```python
from build123d import *

# Parameters (mm, degrees)
F0_R     = 13.7
F1_DEPTH = 2.15
F2_R     = 1
F4_DEPTH = 2.15


with BuildPart() as f1:
    # F0 (on Top) → F1 (new body)
    with BuildSketch(Plane.XY):
        Circle(F0_R)
    extrude(amount=F1_DEPTH)

    # F2
    f2_edges = [f1.edges().sort_by_distance(p)[0] for p in [
        (-13.7, 0, 2.15),
        (-13.7, 0, 0),
    ]]
    fillet(f2_edges, radius=F2_R)

    # F3 (on face) → F4 (cut, through all)
    with BuildSketch(Plane(origin=(0, 0, 0), x_dir=(1, 0, 0), z_dir=(0, 0, -1))):
        Polygon((-3.3669322911, -3.197086975), (-2.673119963, -3.197086975), (-4.7889700387, -0.3285892857), (-2.749716844, 1.8749586682), (-3.4468594713, 1.8749586682), (-5.7469861014, -0.6405273085), (-5.7469861014, 1.8749586682), (-6.3364490553, 1.8749586682), (-6.3364490553, -3.197086975), (-5.7469861014, -3.197086975), (-5.7469861014, -1.2088983676), (-5.2152483331, -0.7371059845), align=None)
        with BuildLine():
            Line((1.1957695829, 0.0513130465), (0.6036887334, 0.1377061204))
            add(Edge.make_bspline(
                [(0.3380255409, -0.3335847345), (0.5428237209, -0.1592137126), (0.6036887334, 0.1377061204)],
                knots=[0, 0, 0, 0.7028049152, 0.7028049152, 0.7028049152], degree=2))
            add(Edge.make_bspline(
                [(-0.5772516823, -0.581692023), (0.0466243631, -0.581692023), (0.3380255409, -0.3335847345)],
                knots=[0, 0, 0, 1, 1, 1], degree=2))
            Line((-0.5772516823, -0.581692023), (-1.3865143818, -0.581692023))
            Line((-1.3865143818, -0.581692023), (-1.3865143818, 0.17412538))
            Line((-1.3865143818, 0.17412538), (-1.9759773358, 0.17412538))
            Line((-1.9759773358, 0.17412538), (-1.9759773358, -3.197086975))
            Line((-1.9759773358, -3.197086975), (-1.3865143818, -3.197086975))
            Line((-1.3865143818, -3.197086975), (-1.3865143818, -1.0878974976))
            Line((-1.3865143818, -1.0878974976), (-0.3274792442, -1.0878974976))
            Line((-0.3274792442, -1.0878974976), (0.9002910515, -3.197086975))
            Line((0.9002910515, -3.197086975), (1.5974336788, -3.197086975))
            Line((1.5974336788, -3.197086975), (0.2197999202, -0.9180522397))
            add(Edge.make_bspline(
                [(1.1957695829, 0.0513130465), (1.0276039433, -0.6376501903), (0.2197999202, -0.9180522397)],
                knots=[0.2081762837, 0.2081762837, 0.2081762837, 1, 1, 1], degree=2))
        make_face()
        with BuildLine():
            add(Edge.make_bspline(
                [(0.6149774989, 0.619108323), (0.5639843778, 0.9626327865), (0.3330300921, 1.1356322514)],
                knots=[0.2207931367, 0.2207931367, 0.2207931367, 1, 1, 1], degree=2))
            Line((0.6149774989, 0.619108323), (1.2327357734, 0.619108323))
            add(Edge.make_bspline(
                [(0.7942765278, 1.5175065568), (1.1831529928, 1.2056305376), (1.2327357734, 0.619108323)],
                knots=[0, 0, 0, 0.872497348, 0.872497348, 0.872497348], degree=2))
            add(Edge.make_bspline(
                [(-0.5850223804, 1.8749586682), (0.3485714883, 1.8749586682), (0.7942765278, 1.5175065568)],
                knots=[0, 0, 0, 1, 1, 1], degree=2))
            Line((-0.5850223804, 1.8749586682), (-1.9759773358, 1.8749586682))
            Line((-1.9759773358, 1.8749586682), (-1.9759773358, 0.7536415942))
            Line((-1.9759773358, 0.7536415942), (-1.3865143818, 0.7536415942))
            Line((-1.3865143818, 0.7536415942), (-1.3865143818, 1.3576521964))
            Line((-1.3865143818, 1.3576521964), (-0.6194354719, 1.3576521964))
            add(Edge.make_bspline(
                [(0.3330300921, 1.1356322514), (0.0366334655, 1.3576521964), (-0.6194354719, 1.3576521964)],
                knots=[0, 0, 0, 1, 1, 1], degree=2))
        make_face()
        with BuildLine():
            Line((3.7232746521, 1.896050563), (3.0058799547, 0.0735661382))
            Line((3.0058799547, 0.0735661382), (3.5263660581, -0.0564224731))
            Line((3.5263660581, -0.0564224731), (3.7443665468, 0.5184168044))
            add(Edge.make_bspline(
                [(3.9630561926, 1.2499725231), (3.8864593116, 0.9169426056), (3.7443665468, 0.5184168044)],
                knots=[0, 0, 0, 1, 1, 1], degree=2))
            add(Edge.make_bspline(
                [(4.1983973343, 0.5184168044), (4.0840570627, 0.8170336304), (3.9630561926, 1.2499725231)],
                knots=[0, 0, 0, 1, 1, 1], degree=2))
            Line((4.1983973343, 0.5184168044), (4.3359644272, 0.1522607828))
            Line((4.3359644272, 0.1522607828), (4.810570116, 0.3869358669))
            Line((4.810570116, 0.3869358669), (4.2194892291, 1.896050563))
            Line((4.2194892291, 1.896050563), (3.7232746521, 1.896050563))
        make_face()
        Polygon((3.3957695214, -0.40078876), (2.8680717842, -0.2765246073), (1.7184345488, -3.197086975), (2.3156682008, -3.197086975), (2.9395442462, -1.5841120746), (4.9721368426, -1.5841120746), (5.6037835861, -3.197086975), (6.2143384348, -3.197086975), (4.9638303876, -0.0043596959), (4.5097831967, -0.3103846639), (4.788970388, -1.0534844061), (3.1482429945, -1.0534844061), align=None)
    extrude(amount=-F4_DEPTH, mode=Mode.SUBTRACT)


solid = f1.part
```
Geometry: final body of the model. Coordinates: model frame, mm. A direction names the side the tool comes from. Give positions to 0.01 mm unless a question says otherwise; leave off trailing zeros.
1. Pin query (flat end, axial travel): P1, Ø0.5, axis at x = -6, z = 1.5, coming from the +Y side; P2, Ø0.8, axis at x = -1, z = 1, coming from the -Y side; P3, Ø0.7, axis at x = -1, z = 1, coming from the +Y side. Return the tip coordinate at first contact, or that it passes through.
2. Line query: probe 1 along Y at (x, z) = (1, 1.15); probe 2 along X at (y, z) = (1.25, 1.2); probe 3 along Y at (x, z) = (-0.75, 1.3). Output: solid intervals per line, ascending.
3. Reachability of faces 3 (the flat face through (-4.304, 1.95, 1.06)), 4 (the flat face through (0, 0, 2.15)) from +Z, -Z, +X, -X, +Y, -Y: full face, straight path, thin tool, end or side. Return the list, or none.
4. Draft query along Y for faces 1 (the flat face through (0, 0, 0)), 2 (the flat face through (-1, -1.875, 1)). Return one class per face: released by +Y, released by -Y, zero draft, split by the parting line, or undercut.
Computed:
1. P1: stops at y = 12.39
1. P2: stops at y = -13.69
1. P3: stops at y = 13.68
2. probe 1: y = -13.66 to -1.3, -0.62 to -0.08, 0.38 to 2.21, 3.2 to 13.66
2. probe 2: x = -13.64 to -6.34, -5.75 to -4.83, -4.11 to -1.98, -1.39 to -0.23, 0.42 to 2.48, 5.45 to 13.64
2. probe 3: y = -13.67 to -1.87, -1.36 to 0.58, 1.09 to 13.67
3. face 3: +Z, -Z
3. face 4: +Z, +X, -X, +Y, -Y
4. face 1: zero draft
4. face 2: undercut
